Could you check a few things on this model? Use its own coordinates, in mm. A direction names the side the tool comes from. Coordinates: 2 decimals unless noted, no trailing zeros. Loops run counter-clockwise (first coordinate to the right, second up) from the corner with the lowest first, then second, coordinate; pieces in that order, holes last. Notation, with made-up numbers: (57.5, 83.5) - (62.5, 83.5) arc R20 ccw to (62.5, 97.5) - close; hole circle Ø11 at (58.5, 75). An arc over 180 degrees is marked (long way). One line per item, written item: value. Start each with the question number.
(1) If we section it at B-B on x = 35.5: Write out the boundary of the cut face in (y, z), then the cut area to 3 significant figures.
(2) I'm going to push flat-ended pins straight in: P1, Ø4, axis at y = 76.5, z = -7.5, coming from the -X side; P2, Ø8, axis at x = 50.5, y = 92.5, coming from the +Z side; P3, Ø17.5, axis at x = 35.5, y = 58.5, coming from the -Z side. Where does each tip first touch, or does it pass through?
(3) On a 3-axis mill with a long thin cutter (end or side, diameter ignored), from which of +Z, -Z, +X, -X, +Y, -Y can I reach the whole of each face in a straight line? I mean faces 1 (the face through (40, 55, -6)), 2 (the face through (51, 51, -8)), 3 (the face through (29, 54, -9)), 4 (the face through (40, 55, -11)). Say none if no direction works.
(4) If I drill on line 1 along Y through (x, z) = (61, -63.5); line 2 along Z through (x, y) = (42.5, 88.5), over which ranges is the centre line in solid material (lowest first)? Write a range as from..to.
(5) If we section it at A-A on y = 48: Write out the boundary of the cut face in (x, z), then the cut area to 3 significant figures.
(6) If we section it at C-C on z = -28.5: Write out the boundary of the cut face in (x, y), then the cut area to 3 significant figures.
Autodesk Inventor part; units mm, degrees
ref_plane "YZ Plane" through (0, 0, 0) normal (1, 0, 0) x (0, 1, 0)
ref_plane "XZ Plane" through (0, 0, 0) normal (0, 1, 0) x (-1, 0, 0)
ref_plane "XY Plane" through (0, 0, 0) normal (0, 0, 1) x (1, 0, 0)
sketch "Sketch1" plane through (0, 0, 0) normal (0, 1, 0) x (-1, 0, 0)
  line L0 (0, 0) -> (-100, 0)
  line L1 (-100, 0) -> (-100, -100)
  line L2 (-100, -100) -> (0, -100)
  line L3 (0, -100) -> (0, 0)
  dimension "d0" = 100
  dimension "d1" = 100
extrude "Extrusion1" add sketch "Sketch1" along normal blind 6
fillet "Fillet1" radius 16.75 4 edges at (100, 3, 0) (100, 3, -100) (0, 3, 0) (0, 3, -100)
sketch "Sketch2" plane through (0, 6, 0) normal (0, 1, 0) x (1, 0, 0)
  line L0 (16.75, 0) -> (83.25, 0)
  line L1 (40, 6) -> (51, 6)
  line L2 (51, 6) -> (51, 11)
  line L3 (51, 11) -> (29, 11)
  line L4 (29, 11) -> (29, 6)
  line L5 (29, 6) -> (40, 6)
  point P0 (0, 0)
extrude "Extrusion2" add sketch "Sketch2" along normal blind 100
sketch "Sketch3" plane through (29, 6, -6) normal (0, 0, 1) x (1, 0, 0)
  line L0 (0, 100) -> (22, 100)
  line L1 (0, 100) -> (22, 91.9927)
  line L2 (22, 0) -> (22, 100)
  line L3 (0, 100) -> (23.4119, 100) construction
  line L4 (22, 91.9927) -> (22, 100)
  line L5 (22, 100) -> (0, 100)
  point P0 (-29, -6)
  dimension "d12" = 20
extrude "Extrusion3" cut sketch "Sketch3" against normal blind 10
fillet "Fillet2" radius 2 2 edges at (29, 106, -8.5) (51, 97.9927, -8.5)
sketch "Sketch4" plane through (51, 6, -11) normal (0, 0, -1) x (-1, 0, 0)
  point P0 (51, -6)
sketch "Sketch5" plane through (29, 6, -6) normal (0, 0, 1) x (1, 0, 0)
  line L0 (0, 99.0231) -> (22, 99.0231)
  point P0 (-29, -6)
properties part number "SmartWatch_Base"
Values:
1. outline: (0, -100) - (6, -100) - (6, -11) - (103.63, -11) - (103.63, -6) - (6, -6) - (6, 0) - (0, 0) - close
1. area: 1,090 mm2
2. P1: stops at x = 29
2. P2: stops at z = -6
2. P3: stops at z = -11
3. face 1: +Z, +X, -X, +Y
3. face 2: +Z, -Z, +X, +Y
3. face 3: +Z, -Z, -X, +Y
3. face 4: -Z, +X, -X, +Y
4. line 1: y = 0..6
4. line 2: z = -11..-6
5. outline: (29, -11) - (51, -11) - (51, -6) - (29, -6) - close
5. area: 110 mm2
6. outline: (0, 0) - (100, 0) - (100, 6) - (0, 6) - close
6. area: 600 mm2
